```python
from build123d import *

# Parameters (mm, degrees)
SKETCH1_R                = 4
BOSS_EXTRUDE1_DEPTH      = 20
BOSS_EXTRUDE1_DEPTH_BACK = 10
CHAMFER1_SIZE            = 0.5
CUT_EXTRUDE1_DEPTH       = 12
SKETCH3_W                = 1.701892275
SKETCH3_H                = 0.6


with BuildPart() as part:
    # Sketch1 → Boss-Extrude1 (new body, two sides)
    with BuildSketch(Plane(origin=(0, 0, 0), x_dir=(1, 0, 0), z_dir=(0, 1, 0))) as boss_extrude1_sk:
        Circle(SKETCH1_R)
    extrude(amount=BOSS_EXTRUDE1_DEPTH)
    extrude(boss_extrude1_sk.sketch, amount=-BOSS_EXTRUDE1_DEPTH_BACK)

    # Chamfer1
    chamfer1_edges = [part.edges().sort_by_distance(p)[0] for p in [
        (-4, 20, 0),
    ]]
    chamfer(chamfer1_edges, length=CHAMFER1_SIZE)

    # Sketch2 → Cut-Extrude1 (cut)
    with BuildSketch(Plane(origin=(0, 20, 0), x_dir=(1, 0, 0), z_dir=(0, 1, 0))):
        with BuildLine():
            Line((-2.645751311, 3), (2.645751311, 3))
            ThreePointArc((2.645751311, 3), (0, 4), (-2.645751311, 3))
        make_face()
    extrude(amount=-CUT_EXTRUDE1_DEPTH, mode=Mode.SUBTRACT)

    # Sketch3 → Cut-Revolve1 (revolve, cut)
    with BuildSketch(Plane(origin=(0, 0, 0), x_dir=(0, 0, -1), z_dir=(1, 0, 0))):
        with Locations((4.050946138, 0.3)):
            Rectangle(SKETCH3_W, SKETCH3_H)
    revolve(axis=Axis((0, 0, 0), (0, 1, 0)), mode=Mode.SUBTRACT)


solid = part.part
```
The model under review builds one solid part; all positions refer to its coordinate system, in mm. A direction names the side the tool comes from. Round coordinates to 2 decimals unless told otherwise and drop trailing zeros. Order: outer loops, then holes, each group sorted by start corner. A loop starts at its lowest first (then second) coordinate and runs counter-clockwise, first axis right, second up. Notation, with made-up numbers: (38, -1) -> (65, -1) arc R9 ccw to (65, 8) -> close; hole circle Ø4 at (-13, 80.25). An arc over 180 degrees is marked (long way). One line per item, written item: value. Start each with the question number.
Q1. Mouldability with a two-part tool opening along Y and no side actions: class faces 1 (the face through (-0.132, 19.865, 3.633)), 2 (the face through (0, 14, -3)), 3 (the face through (3.124, 0.304, 0.694)) as released by +Y, released by -Y, zero draft, split by the parting line, or undercut.
Q2. Take a section at A-A (x = 0). Write out the cut boundary in (y, z).
Q3. Take a section at B-B (y = -1). Write out the cut boundary in (x, z), and give its area (3 significant figures).
Q4. Machinability: for faces 4 (the face through (0, 8, -3.4)), 5 (the face through (-3, 0, -2)), 6 (the face through (-0.867, -4.93, 3.905)), which of the approach directions +Z, -Z, +X, -X, +Y, -Y give a long, thin tool a straight path to every point of the face, cutting with its end or side? Answer none if there is none.
Q5. Wall thickness on line 1 (X direction, y = -5, z = 3); line 2 (Z direction, x = 3.5, y = 11): over which ranges is each line inside the solid? List them lowest first.
Q6. Clearance check with flat-ended pins moving along their axes: pin 1 Ø2 at (x, y) = (-2.5, 6) entering from -Z; pin 2 Ø4 at (x, y) = (-0.5, 13) entering from -Z; pin 3 Ø1 at (x, y) = (1, 7) entering from +Z. State where each tip first meets the part, or that it passes through.
Reported:
1. face 1: released by +Y
1. face 2: zero draft
1. face 3: undercut
2. outline: (-10, -4) -> (0, -4) -> (0, -3.2) -> (0.6, -3.2) -> (0.6, -4) -> (8, -4) -> (8, -3) -> (20, -3) -> (20, 3.5) -> (19.5, 4) -> (0.6, 4) -> (0.6, 3.2) -> (0, 3.2) -> (0, 4) -> (-10, 4) -> close
3. outline: circle Ø8 at (0, 0)
3. area: 50.3 mm2
4. face 4: -Z, +X, -X, +Y
4. face 5: none
4. face 6: +Y, -Y
5. line 1: x = -2.65 to 2.65
5. line 2: z = -1.94 to 1.94
6. pin 1: stops at z = -3.71
6. pin 2: stops at z = -3
6. pin 3: stops at z = 3.97
